```python
from build123d import *

# Parameters (mm, degrees)
F1_DEPTH = 9.525
F2_R     = 1.89865
F3_DEPTH = 1.5885
F5_DEPTH = 9.525


with BuildPart() as f1:
    # F0 (on Front) → F1 (new body)
    with BuildSketch(Plane.XZ):
        with BuildLine():
            ThreePointArc((13.0392482051, -25.4265339999), (0, -28.575), (-13.0392482051, -25.4265339999))
            Line((-13.0392482051, -25.4265339999), (-13.7636508831, -26.8391192221))
            ThreePointArc((-13.7636508831, -26.8391192221), (0, -30.1625), (13.7636508831, -26.8391192221))
            Line((13.7636508831, -26.8391192221), (13.0392482051, -25.4265339999))
        make_face()
        with BuildLine():
            Line((15.157159657, -26.0775174697), (14.4316955802, -24.66286252))
            ThreePointArc((14.4316955802, -24.66286252), (13.7407782402, -25.0543736372), (13.0392482051, -25.4265339999))
            Line((13.0392482051, -25.4265339999), (13.7636508831, -26.8391192221))
            ThreePointArc((13.7636508831, -26.8391192221), (14.4654184136, -26.4674909345), (15.157159657, -26.0775174697))
        make_face()
        with BuildLine():
            Line((16.844971211, -29.36875), (15.157159657, -26.0775174697))
            ThreePointArc((15.157159657, -26.0775174697), (14.4654184136, -26.4674909345), (13.7636508831, -26.8391192221))
            Line((13.7636508831, -26.8391192221), (15.875, -30.95625))
            Line((15.875, -30.95625), (26.369971211, -30.95625))
            Line((26.369971211, -30.95625), (26.369971211, -29.36875))
            Line((26.369971211, -29.36875), (16.844971211, -29.36875))
        make_face()
        with BuildLine():
            ThreePointArc((-13.0392482051, -25.4265339999), (-13.7407782402, -25.0543736372), (-14.4316955802, -24.66286252))
            Line((-14.4316955802, -24.66286252), (-15.157159657, -26.0775174697))
            ThreePointArc((-15.157159657, -26.0775174697), (-14.4654184136, -26.4674909345), (-13.7636508831, -26.8391192221))
            Line((-13.7636508831, -26.8391192221), (-13.0392482051, -25.4265339999))
        make_face()
        with BuildLine():
            ThreePointArc((-13.7636508831, -26.8391192221), (-14.4654184136, -26.4674909345), (-15.157159657, -26.0775174697))
            Line((-15.157159657, -26.0775174697), (-16.844971211, -29.36875))
            Line((-16.844971211, -29.36875), (-26.369971211, -29.36875))
            Line((-26.369971211, -29.36875), (-26.369971211, -30.95625))
            Line((-26.369971211, -30.95625), (-15.875, -30.95625))
            Line((-15.875, -30.95625), (-13.7636508831, -26.8391192221))
        make_face()
    extrude(amount=F1_DEPTH)

    # F2 (on face) → F3 (cut, through all)
    with BuildSketch(Plane.XY.offset(-29.36875)):
        with Locations((21.607471211, -4.7625)):
            Circle(F2_R)
        with Locations((-21.607471211, -4.7625)):
            Circle(F2_R)
    extrude(amount=-F3_DEPTH, mode=Mode.SUBTRACT)

    # F4 (on face) → F5 (join, through all)
    with BuildSketch(Plane.XZ.offset(9.525)):
        with BuildLine():
            Line((-13.7636508831, -26.8391192221), (-15.875, -30.95625))
            Line((-15.875, -30.95625), (15.875, -30.95625))
            Line((15.875, -30.95625), (13.7636508831, -26.8391192221))
            ThreePointArc((13.7636508831, -26.8391192221), (0, -30.1625), (-13.7636508831, -26.8391192221))
        make_face()
    extrude(amount=-F5_DEPTH)


solid = f1.part
```
CAD build for the part. Positions are in the model's coordinates, mm. A direction names the side the tool comes from. Coordinates: 2 decimals unless noted, no trailing zeros. Loops run counter-clockwise (first coordinate to the right, second up) from the corner with the lowest first, then second, coordinate; pieces in that order, holes last. Notation, with made-up numbers: (62, 35.5) - (99, 35.5) arc R32 cw to (99, 62.5) - close; hole circle Ø1 at (-14.75, -13.5). An arc over 180 degrees is marked (long way). Return JSON: item names as keys, results as strings.
1. Band-saw the part on A-A (z = -27). Give the cut face in (x, y) (3 decimals), and give its area (3 significant figures).
Result:
{"outline": "(-15.63, -9.525) - (-9.356, -9.525) - (-9.356, 0) - (-15.63, 0) - close; (9.356, -9.525) - (15.63, -9.525) - (15.63, 0) - (9.356, 0) - close", "area": "120 mm2"}
2. 3-axis set-ups, long thin cutter, end or side, ignore diameter. For faces 1 (the flat face through (-24, -5, -29.369)), 2 (the flat face through (-26.37, -5, -30)), 3 (the flat face through (24, -5, -29.369)): which of +Z, -Z, +X, -X, +Y, -Y reach the whole face in a straight line?
Result:
{"face 1": "+Z, -X, +Y, -Y", "face 2": "+Z, -Z, -X, +Y, -Y", "face 3": "+Z, +X, +Y, -Y"}
3. Drop flat-ended pins along their axis: pin 1 (4 mm diameter, centred on x = 11, y = -3, fed in from +Z); pin 2 (5 mm diameter, centred on x = 23, y = -7, fed in from +Z). Give the stop position or say it passes through.
Result:
{"pin 1": "stops at z = -25.45", "pin 2": "stops at z = -29.37"}
4. Mould opens along Y. For faces 4 (the flat face through (0, 0, -29)), 5 (the flat face through (0, -9.525, -29)), 6 (the cylindrical face through (21.196, -6.616, -30.151)) say: released by +Y, released by -Y, zero draft, split by the parting line, or undercut.
Result:
{"face 4": "released by +Y", "face 5": "released by -Y", "face 6": "undercut"}
5. Band-saw the part on C-C (x = -21). Give the cut face in (y, z) (3 decimals).
Result:
{"outline": "(-9.525, -30.956) - (-6.561, -30.956) - (-6.561, -29.369) - (-9.525, -29.369) - close; (-2.964, -30.956) - (0, -30.956) - (0, -29.369) - (-2.964, -29.369) - close"}
6. Band-saw the part on B-B (y = -4). Give the cut face in (x, z) (3 decimals), and give its area (3 significant figures).
Result:
{"outline": "(-26.37, -30.956) - (-23.346, -30.956) - (-23.346, -29.369) - (-26.37, -29.369) - close; (-19.869, -30.956) - (19.869, -30.956) - (19.869, -29.369) - (16.845, -29.369) - (14.432, -24.663) arc R28.575 cw to (-14.432, -24.663) - (-16.845, -29.369) - (-19.869, -29.369) - close; (23.346, -30.956) - (26.37, -30.956) - (26.37, -29.369) - (23.346, -29.369) - close", "area": "143 mm2"}
7. Band-saw the part on D-D (y = -9). Give the cut face in (x, z) (3 decimals), and give its area (3 significant figures).
Result:
{"outline": "(-26.37, -30.956) - (26.37, -30.956) - (26.37, -29.369) - (16.845, -29.369) - (14.432, -24.663) arc R28.575 cw to (-14.432, -24.663) - (-16.845, -29.369) - (-26.37, -29.369) - close", "area": "155 mm2"}
8. Probe L1, parallel to Z at x = 0.5, y = -2.5; L2, parallel to X at y = -3.75, z = -30.25; L3, parallel to Z at x = -17, y = -6.75. List the from-to ranges inside material, lowest first. Write a range as from..to.
Result:
{"L1": "z = -30.96..-28.57", "L2": "x = -26.37..-23.21, -20..20, 23.21..26.37", "L3": "z = -30.96..-29.37"}
